from build123d import *

# Parameters (mm, degrees)
SKETCH029_R     = 22.75
SKETCH029_R_2   = 14
PAD009_DEPTH    = 3.5
CHAMFER007_SIZE = 1
SKETCH026_R     = 16
SKETCH026_R_2   = 14
PAD010_DEPTH    = 25
SKETCH030_R     = 0.95
POCKET012_DEPTH = 3
SKETCH032_R     = 1.65
POCKET014_DEPTH = 1.5
CHAMFER011_SIZE = 1.5


with BuildPart() as part:
    # Sketch029 → Pad009 (new body)
    with BuildSketch(Plane.XY):
        Circle(SKETCH029_R)
        Circle(SKETCH029_R_2, mode=Mode.SUBTRACT)
    extrude(amount=-PAD009_DEPTH)

    # Chamfer007
    chamfer007_edges = [part.edges().sort_by_distance(p)[0] for p in [
        (-22.75, 0, -3.5),
    ]]
    chamfer(chamfer007_edges, length=CHAMFER007_SIZE)

    # Sketch026 → Pad010 (join)
    with BuildSketch(Plane.XY):
        Circle(SKETCH026_R)
        Circle(SKETCH026_R_2, mode=Mode.SUBTRACT)
    extrude(amount=-PAD010_DEPTH)

    # Sketch030 → Pocket012 (cut)
    with BuildSketch(Plane.XY):
        with Locations((-19.5, 0)):
            Circle(SKETCH030_R)
        with Locations((0, -19.5)):
            Circle(SKETCH030_R)
        with Locations((19.5, 0)):
            Circle(SKETCH030_R)
        with Locations((0, 19.5)):
            Circle(SKETCH030_R)
    extrude(amount=-POCKET012_DEPTH, mode=Mode.SUBTRACT)

    # Sketch032 → Pocket014 (cut)
    with BuildSketch(Plane.XY.offset(-3.5)):
        with Locations((-19.5, 0)):
            Circle(SKETCH032_R)
        with Locations((0, -19.5)):
            Circle(SKETCH032_R)
        with Locations((19.5, 0)):
            Circle(SKETCH032_R)
        with Locations((0, 19.5)):
            Circle(SKETCH032_R)
    extrude(amount=POCKET014_DEPTH, mode=Mode.SUBTRACT)

    # Chamfer011
    chamfer011_edges = [part.edges().sort_by_distance(p)[0] for p in [
        (-16, 0, -25),
    ]]
    chamfer(chamfer011_edges, length=CHAMFER011_SIZE)


with BuildPart() as part_1:
    # Body006 placement: moved
    add(part.part.moved(Location((0, 0, -1))))


solid = part_1.part
Verification items for the finished model (mm, model axes). A direction names the side the tool comes from. Give positions to 0.01 mm unless a question says otherwise; leave off trailing zeros. Write each loop counter-clockwise with the first axis right and the second up, starting at its lowest first coordinate (ties: lowest second). Pieces come first, ordered by that corner, then holes. Notation, with made-up numbers: M -14,-28 L 12,-28 A21 cw 12,9 Z; hole C 51,78.25 d5. An arc over 180 degrees is marked long. Put each result on its own line as item: value. Start each with the question number.
1. Section check C-C (z = -23). Record the cut outline in (x, y), and give its area (3 significant figures).
2. Scan lines: line 1 along Y through (x, z) = (0, -1.7); line 2 along Y through (x, z) = (0, -3.45); line 3 along Y through (x, z) = (0, -11.25). Record each from-to range of solid material in increasing order. Write a range as [from, to].
3. Go/stop test with flat-tipped pins: pin 1 Ø1 at (x, y) = (0, 20) entering from -Z; pin 2 Ø2 at (y, z) = (-11.5, -8) entering from +X; pin 3 Ø22.5 at (x, y) = (0, 0) entering from -Z; pin 4 Ø4 at (y, z) = (-6.5, -13.5) entering from +X. Record where each tip stops, or that it passes through.
4. Section check A-A (x = 0). Give the number of separate pieces and of enclosed holes in the cut face, and give its area (4 significant figures).
5. Set-up check for faces 1 (the face through (-0.206, 18.573, -1.986)), 2 (the face through (-19, -1, -3)): record each of +Z, -Z, +X, -X, +Y, -Y from which the full face is reachable in a straight line by a thin tool's end or side.
6. Draft check along Y on faces 3 (the face through (12.932, -5.362, -13.325)), 4 (the face through (9.8, 10.4, -1)), 5 (the face through (-18.054, -13.843, -2.232)). Enter one of: +Y half, -Y half, draft (parallel to the pull), parting line (faces both ways), or undercut.
7. Section check B-B (z = -2.25). Record the cut outline in (x, y), and give its area (3 significant figures).
Answer list:
1. outline: C 0,0 d32; hole C 0,0 d28
1. area: 188 mm2
2. line 1: [-22.75, -20.45], [-18.55, -14], [14, 18.55], [20.45, 22.75]
2. line 2: [-22.75, -21.15], [-17.85, -14], [14, 17.85], [21.15, 22.75]
2. line 3: [-16, -14], [14, 16]
3. pin 1: z = -3
3. pin 2: x = 12.07
3. pin 3: through
3. pin 4: x = 15.35
4. separate pieces: 4
4. enclosed holes: 0
4. area: 126.5 mm2
5. face 1: +Z, -Z
5. face 2: -Z
6. face 3: undercut
6. face 4: draft
6. face 5: parting line
7. outline: C 0,0 d45.5; hole C -19.5,0 d1.9; hole C 0,0 d28; hole C 0,-19.5 d1.9; hole C 0,19.5 d1.9; hole C 19.5,0 d1.9
7. area: 999 mm2
